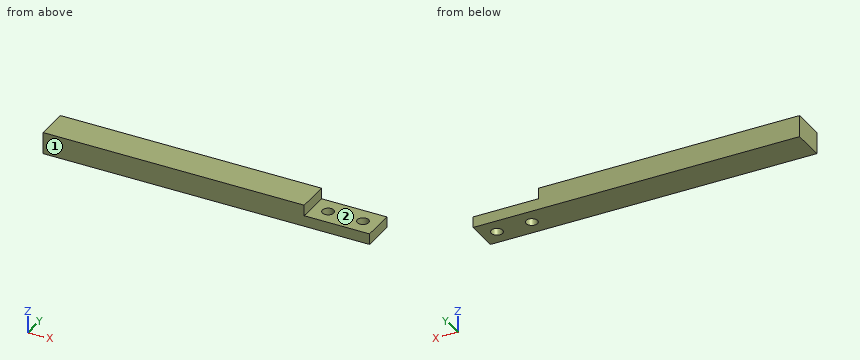
```python
from build123d import *

# Parameters (mm, degrees)
PAD_DEPTH    = 15
SKETCH001_R  = 2.625
POCKET_DEPTH = 5


with BuildPart() as part:
    # Sketch → Pad (new body)
    with BuildSketch(Plane.XZ):
        Polygon((-68.87526, -5.227487), (-68.87526, 4.772513), (51.12474, 4.772513), (51.12474, -0.227487), (81.12474, -0.227487), (81.12474, -5.227487), align=None)
    extrude(amount=PAD_DEPTH)

    # Sketch001 (on Face4 of Pad) → Pocket (cut)
    with BuildSketch(Plane(origin=(0, 0, -0.227487), x_dir=(-1, 0, 0), z_dir=(0, 0, 1))):
        with Locations((-74.12474, 7.5)):
            Circle(SKETCH001_R)
        with Locations((-58.12474, 7.5)):
            Circle(SKETCH001_R)
    extrude(amount=-POCKET_DEPTH, mode=Mode.SUBTRACT)


solid = part.part
```
Read the model definition and answer for the solid it produces. Units are mm, in the model's axes. Face numbers are marked on the shaded views. A direction names the side the tool comes from. Give positions to 0.01 mm unless a question says otherwise; leave off trailing zeros. Order: outer loops, then holes, each group sorted by start corner. A loop starts at its lowest first (then second) coordinate and runs counter-clockwise, first axis right, second up. Notation, with made-up numbers: (-20, 42.5) -> (27, 42.5) arc R27 ccw to (27, 68.5) -> close; hole circle Ø2 at (20, 85.5). An arc over 180 degrees is marked (long way). One line per item, written item: value. Start each with the question number.
(1) The part is cut by section C-C (x = 64). Determine the outline of the cut face in (y, z), and give its area (3 significant figures).
(2) The part is cut by section D-D (y = -13.75). Determine the outline of the cut face in (x, z), and give its area (3 significant figures).
(3) A tool of negligible diameter and unlimited length cuts with its end or side. For the marked faces 1 and 2, from which of +Z, -Z, +X, -X, +Y, -Y can it reach the whole face along a straight path? Write none if from no direction.
(4) The part is cut by section B-B (z = -3.25). Determine the outline of the cut face in (x, y) (3 decimals), and give its area (3 significant figures).
(5) Straight lines are drawn through the part: L1, parallel to X at y = -7.5, z = -3.4; L2, parallel to X at y = -8.75, z = 2; L3, parallel to Z at x = 57.5, y = -11. For each, find the intervals that lie inside material, in ascending order.
(6) Flat-ended cylindrical pins translate along their axes: P1, Ø6, axis at x = 74.12, y = -7.5, coming from the +Z side; P2, Ø5.5, axis at y = -5.5, z = 3, coming from the +X side. Find the tip coordinate at first contact, or state that the pin passes through.
(7) The part is cut by section A-A (y = -7.5). Determine the outline of the cut face in (x, z).
Taken from the geometry:
1. outline: (-15, -5.23) -> (0, -5.23) -> (0, -0.23) -> (-15, -0.23) -> close
1. area: 75.0 mm^2
2. outline: (-68.88, -5.23) -> (81.12, -5.23) -> (81.12, -0.23) -> (51.12, -0.23) -> (51.12, 4.77) -> (-68.88, 4.77) -> close
2. area: 1,350 mm^2
3. face 1: +Z, -Z, +X, -X, -Y
3. face 2: +Z, +X, +Y, -Y
4. outline: (-68.875, -15) -> (81.125, -15) -> (81.125, 0) -> (-68.875, 0) -> close; hole circle Ø5.25 at (58.125, -7.5); hole circle Ø5.25 at (74.125, -7.5)
4. area: 2,210 mm^2
5. L1: -68.88 to 55.5, 60.75 to 71.5, 76.75 to 81.12
5. L2: -68.88 to 51.12
5. L3: -5.23 to -0.23
6. P1: z = -0.23
6. P2: x = 51.12
7. outline: (-68.88, -5.23) -> (55.5, -5.23) -> (55.5, -0.23) -> (51.12, -0.23) -> (51.12, 4.77) -> (-68.88, 4.77) -> close; (60.75, -5.23) -> (71.5, -5.23) -> (71.5, -0.23) -> (60.75, -0.23) -> close; (76.75, -5.23) -> (81.12, -5.23) -> (81.12, -0.23) -> (76.75, -0.23) -> close
